Can you work these out from the model? Positions are in its coordinate system, mm. Round coordinates to 2 decimals unless told otherwise and drop trailing zeros. Use a Markdown table: item, result. Add a question column.
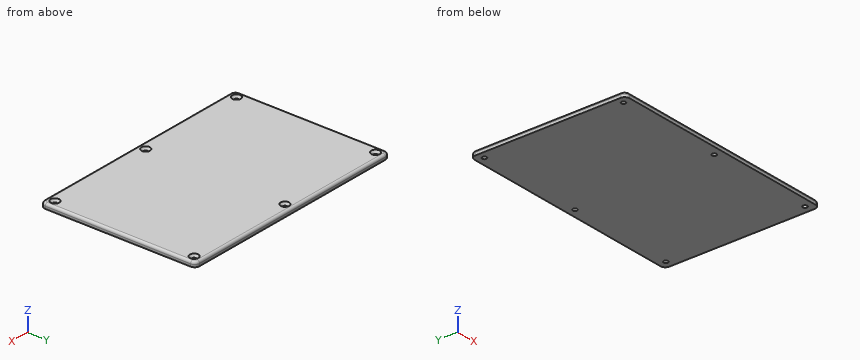
```python
from build123d import *

# Parameters (mm, degrees)
SKETCH3_W           = 191
SKETCH3_H           = 127
BOSS_EXTRUDE3_DEPTH = 4
SKETCH6_R           = 4
BOSS_EXTRUDE4_DEPTH = 0.001
HOLE1_D             = 3.6
HOLE1_DEPTH         = 5
HOLE1_CSINK_D       = 7.1
HOLE1_CSINK_ANGLE   = 82
FILLET1_R           = 4
FILLET2_R           = 2


with BuildPart() as part:
    # Sketch3 → Boss-Extrude3 (new body)
    with BuildSketch(Plane.XY):
        Rectangle(SKETCH3_W, SKETCH3_H)
    extrude(amount=BOSS_EXTRUDE3_DEPTH)

    # Sketch6 → Boss-Extrude4 (add)
    with BuildSketch(Plane.XY):
        with Locations((-89.294075307, 57.128381867)):
            Circle(SKETCH6_R)
        with Locations((89.301830171, 57.128381867)):
            Circle(SKETCH6_R)
        with Locations((89.301830171, -56.852590264)):
            Circle(SKETCH6_R)
        with Locations((-89.294075307, -56.852590264)):
            Circle(SKETCH6_R)
        with Locations((0, -56.852590264)):
            Circle(SKETCH6_R)
        with Locations((0, 57.128381867)):
            Circle(SKETCH6_R)
    extrude(amount=BOSS_EXTRUDE4_DEPTH)

    # Hole1
    with Locations(Plane(origin=(-89.358562902, 57.095579806, 4), x_dir=(1, 0, 0), z_dir=(0, 0, 1))):
        with Locations((0, 0), (89.166832603, 0.030108388), (178.563780061, 0.049936098), (178.506385813, -113.977594328), (89.197749936, -113.952124174), (-0.085769967, -113.957972021)):
            CounterSinkHole(HOLE1_D / 2, HOLE1_CSINK_D / 2, depth=HOLE1_DEPTH, counter_sink_angle=HOLE1_CSINK_ANGLE)

    # Fillet1
    fillet1_edges = [part.edges().sort_by_distance(p)[0] for p in [
        (95.5, -63.5, 2),
        (-95.5, -63.5, 2),
        (-95.5, 63.5, 2),
        (95.5, 63.5, 2),
    ]]
    fillet(fillet1_edges, radius=FILLET1_R)

    # Fillet2
    fillet2_edges = [part.edges().sort_by_distance(p)[0] for p in [
        (-95.5, 0, 4),
        (0, 63.5, 4),
        (95.5, 0, 4),
        (0, -63.5, 4),
        (94.328427125, -62.328427125, 4),
        (94.328427125, 62.328427125, 4),
        (-94.328427125, -62.328427125, 4),
        (-94.328427125, 62.328427125, 4),
    ]]
    fillet(fillet2_edges, radius=FILLET2_R)


solid = part.part
```
(1) If I drill on probe 1 along X at (y, z) = (-56, 3.7); probe 2 along Y at (x, z) = (-82, 2.2); probe 3 along X at (y, z) = (-48, 2.4), over which ranges is the centre line in solid material (lowest first)? Write a range as [from, to].
(2) I'm going to push flat-ended pins straight in: pin 1 (4 mm diameter, centred on x = -89.44, y = -56.86, fed in from +Z); pin 2 (4.5 mm diameter, centred on x = -89.36, y = 57.1, fed in from +Z); pin 3 (1 mm diameter, centred on y = -33.5, z = 3.5, fed in from -X). Where does each tip first touch, or does it pass through?
(3) Suppose I cut it at A-A on z = 3.4. Count the separate pieces of the cut face and the enclosed holes in it, and give its area (3 significant figures).
Results below:
| question | item | result |
|---|---|---|
| 1 | probe 1 | x = [-94.55, -92.62], [-86.27, -3.34], [3.01, 85.98], [92.32, 94.55] |
| 1 | probe 2 | y = [-63.49, 63.49] |
| 1 | probe 3 | x = [-95.46, 95.46] |
| 2 | pin 1 | stops at z = 2.22 |
| 2 | pin 2 | stops at z = 2.51 |
| 2 | pin 3 | stops at x = -95.23 |
| 3 | separate pieces | 1 |
| 3 | enclosed holes | 6 |
| 3 | area | 23,700 mm² |
